Autodesk Inventor part; units mm, degrees
ref_plane "YZ Plane" through (0, 0, 0) normal (1, 0, 0) x (0, 1, 0)
ref_plane "XZ Plane" through (0, 0, 0) normal (0, 1, 0) x (-1, 0, 0)
ref_plane "XY Plane" through (0, 0, 0) normal (0, 0, 1) x (1, 0, 0)
sketch "Sketch1" plane through (0, 0, 0) normal (0, 0, 1) x (1, 0, 0)
  line L0 (0, 0) -> (0, 9.525) construction
  line L1 (0, 6.35) -> (1.5875, 6.35)
  line L2 (1.5875, 6.35) -> (1.5875, 9.3918)
  line L3 (0, 6.35) -> (-1.5875, 6.35)
  line L4 (-1.5875, 6.35) -> (-1.5875, 9.3918)
  line L5 (-6.293, 1.8002) -> (-8.9273, 3.3211)
  line L6 (-5.4993, 3.175) -> (-6.293, 1.8002)
  line L7 (-5.4993, 3.175) -> (-4.7055, 4.5498)
  line L8 (-4.7055, 4.5498) -> (-7.3398, 6.0707)
  line L9 (-4.7055, -4.5498) -> (-7.3398, -6.0707)
  line L10 (-5.4993, -3.175) -> (-4.7055, -4.5498)
  line L11 (-5.4993, -3.175) -> (-6.293, -1.8002)
  line L12 (-6.293, -1.8002) -> (-8.9273, -3.3211)
  line L13 (1.5875, -6.35) -> (1.5875, -9.3918)
  line L14 (0, -6.35) -> (1.5875, -6.35)
  line L15 (0, -6.35) -> (-1.5875, -6.35)
  line L16 (-1.5875, -6.35) -> (-1.5875, -9.3918)
  line L17 (6.293, -1.8002) -> (8.9273, -3.3211)
  line L18 (5.4993, -3.175) -> (6.293, -1.8002)
  line L19 (5.4993, -3.175) -> (4.7055, -4.5498)
  line L20 (4.7055, -4.5498) -> (7.3398, -6.0707)
  line L21 (4.7055, 4.5498) -> (7.3398, 6.0707)
  line L22 (5.4993, 3.175) -> (4.7055, 4.5498)
  line L23 (5.4993, 3.175) -> (6.293, 1.8002)
  line L24 (6.293, 1.8002) -> (8.9273, 3.3211)
  arc A0 (-1.5875, 9.3918) -> (-7.3398, 6.0707) centre (0, 0) ccw
  arc A1 (-8.9273, 3.3211) -> (-8.9273, -3.3211) centre (0, 0) ccw
  arc A2 (-7.3398, -6.0707) -> (-1.5875, -9.3918) centre (0, 0) ccw
  arc A3 (1.5875, -9.3918) -> (7.3398, -6.0707) centre (0, 0) ccw
  arc A4 (8.9273, -3.3211) -> (8.9273, 3.3211) centre (0, 0) ccw
  arc A5 (7.3398, 6.0707) -> (1.5875, 9.3918) centre (0, 0) ccw
  dimension "splineDepth" = 3.175
  dimension "splineWidth" = 3.175
  dimension "d6" = 360
extrude "Extrusion1" add sketch "Sketch1" against normal blind 50.8
sketch "Sketch2" plane through (0, 0, -50.8) normal (0, 0, -1) x (-1, 0, 0)
  circle A0 centre (0, 0) radius 6.35
  dimension "innerDiameter" = 12.7
extrude "Extrusion2" add sketch "Sketch2" along normal blind 50.8
sketch "Sketch3" plane through (0, 0, 0) normal (0, 0, 1) x (1, 0, 0)
  circle A0 centre (0, 0) radius 6.35
  dimension "d13" = 12.7
extrude "Extrusion3" add sketch "Sketch3" along normal blind 50.8
equation "\"d13\" = innerDiameter"
properties part number "innerShaft" material "PET Plastic"
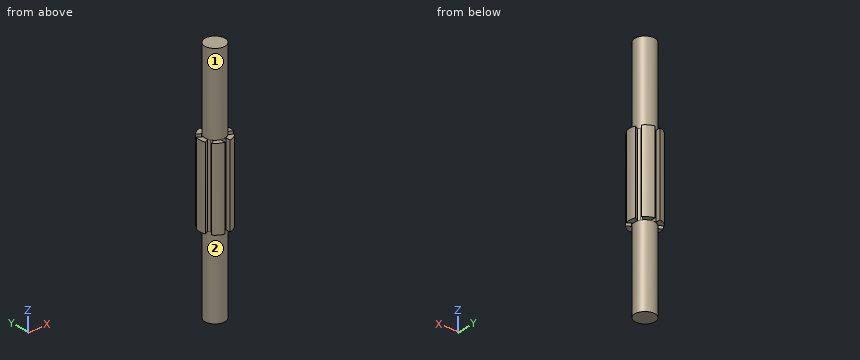
The model under review builds one solid part; all positions refer to its coordinate system, in mm. Face numbers are marked on the shaded views. A direction names the side the tool comes from. Give positions to 0.01 mm unless a question says otherwise; leave off trailing zeros. Loops run counter-clockwise (first coordinate to the right, second up) from the corner with the lowest first, then second, coordinate; pieces in that order, holes last. Notation, with made-up numbers: (66, 16) -> (116, 16) arc R20 ccw to (116, 41) -> close; hole circle Ø7 at (-9, -31). An arc over 180 degrees is marked (long way). Put each result on its own line as item: value. Start each with the question number.
1. We need section B-B on y = 0. State the section outline as (x, z) points, then the cut area to 3 significant figures.
2. Wall thickness on probe 1 along X at (y, z) = (-2.5, -9); probe 2 along Y at (x, z) = (-0.5, -60); probe 3 along Z at (x, y) = (-8, 0): over which ranges is each line inside the solid? List them lowest first.
3. We need section D-D on x = -3.25. State the section outline as (y, z) points.
4. Clearance check with flat-ended pins moving along their axes: P1, Ø1.5, axis at x = 7, y = 4, coming from the -Z side; P2, Ø2.5, axis at y = 8.5, z = -38, coming from the +X side; P3, Ø1, axis at x = -0.5, z = -25.5, coming from the -Y side; P4, Ø2.5, axis at y = 8.5, z = -23.5, coming from the -X side. State where each tip first meets the part, or that it passes through.
5. We need section C-C on y = -8. State the section outline as (x, z) points, then the cut area to 3 significant figures.
6. For the marked faces 1 and 2, list the 3-axis set-ups (+Z, -Z, +X, -X, +Y, -Y) from which the entire face can be reached by the end or side of a thin tool; tool diameter is ignored.
Determined:
1. outline: (-9.53, -50.8) -> (-6.35, -50.8) -> (-6.35, -101.6) -> (6.35, -101.6) -> (6.35, -50.8) -> (9.53, -50.8) -> (9.53, 0) -> (6.35, 0) -> (6.35, 50.8) -> (-6.35, 50.8) -> (-6.35, 0) -> (-9.53, 0) -> close
1. area: 2,260 mm^2
2. probe 1: -9.19 to -7.51, -5.89 to 5.89, 7.51 to 9.19
2. probe 2: -6.33 to 6.33
2. probe 3: -50.8 to 0
3. outline: (-8.95, -50.8) -> (-5.46, -50.8) -> (-5.46, -101.6) -> (5.46, -101.6) -> (5.46, -50.8) -> (8.95, -50.8) -> (8.95, 0) -> (5.46, 0) -> (5.46, 50.8) -> (-5.46, 50.8) -> (-5.46, 0) -> (-8.95, 0) -> close
4. P1: through
4. P2: x = 6.18
4. P3: y = -6.35
4. P4: x = -6.18
5. outline: (-5.17, -50.8) -> (-1.59, -50.8) -> (-1.59, 0) -> (-5.17, 0) -> close; (1.59, -50.8) -> (5.17, -50.8) -> (5.17, 0) -> (1.59, 0) -> close
5. area: 364 mm^2
6. face 1: +Z
6. face 2: -Z
